Check sheet for the modelled part. Datum: model origin and axes. Units: mm. A direction names the side the tool comes from. Give positions to 0.01 mm unless a question says otherwise; leave off trailing zeros. Loops run counter-clockwise (first coordinate to the right, second up) from the corner with the lowest first, then second, coordinate; pieces in that order, holes last. Notation, with made-up numbers: (55, 76) - (100, 76) arc R22 cw to (100, 114) - close; hole circle Ø6 at (-12.5, -30). An arc over 180 degrees is marked (long way). Use one line per item in the form item = value.
from build123d import *

# Parameters (mm, degrees)
SKETCH_3_W          = 10
SKETCH_3_H          = 3
EXTRUDE_1_DEPTH     = 10
EXTRUDE_1_2_DEPTH   = 10
EXTRUDE_1_3_DEPTH   = 10
EXTRUDE_1_4_DEPTH   = 10
SKETCH_4_W          = 65
SKETCH_4_H          = 9
EXTRUDE_2_DEPTH     = 3
SKETCH_5_R          = 2.1
CUT_EXTRUDE_1_DEPTH = 17
SKETCH_7_W          = 65
SKETCH_7_H          = 3
EXTRUDE_3_DEPTH     = 4
SKETCH_8_W          = 65
SKETCH_8_H          = 3
EXTRUDE_4_DEPTH     = 4


with BuildPart() as part:
    # Sketch 3 → Extrude 1 (new body)
    with BuildSketch(Plane(origin=(0, 0, 0), x_dir=(1, 0, 0), z_dir=(0, 1, 0))):
        Rectangle(SKETCH_3_W, SKETCH_3_H)
    extrude(amount=EXTRUDE_1_DEPTH)



with BuildPart() as body_2:
    # Sketch 3 → Extrude 1 2 (new body)
    with BuildSketch(Plane(origin=(0, 0, 0), x_dir=(1, 0, 0), z_dir=(0, 1, 0))):
        with Locations((55, 0)):
            Rectangle(SKETCH_3_W, SKETCH_3_H)
    extrude(amount=EXTRUDE_1_2_DEPTH)


with BuildPart() as body_3:
    # Sketch 3 → Extrude 1 3 (new body)
    with BuildSketch(Plane(origin=(0, 0, 0), x_dir=(1, 0, 0), z_dir=(0, 1, 0))):
        with Locations((0, 6)):
            Rectangle(SKETCH_3_W, SKETCH_3_H)
    extrude(amount=EXTRUDE_1_3_DEPTH)


with BuildPart() as body_4:
    # Sketch 3 → Extrude 1 4 (new body)
    with BuildSketch(Plane(origin=(0, 0, 0), x_dir=(1, 0, 0), z_dir=(0, 1, 0))):
        with Locations((55, 6)):
            Rectangle(SKETCH_3_W, SKETCH_3_H)
    extrude(amount=EXTRUDE_1_4_DEPTH)


with BuildPart() as part_1:
    add(part.part)

    add(body_2.part)  # Extrude 2 merges body 2

    add(body_3.part)  # Extrude 2 merges body 3

    add(body_4.part)  # Extrude 2 merges body 4
    # Sketch 4 → Extrude 2 (add)
    with BuildSketch(Plane(origin=(0, 10, 0), x_dir=(1, 0, 0), z_dir=(0, 1, 0))):
        with Locations((27.5, 3)):
            Rectangle(SKETCH_4_W, SKETCH_4_H)
    extrude(amount=EXTRUDE_2_DEPTH)

    # Sketch 5 → Cut-Extrude 1 (cut)
    with BuildSketch(Plane.XY.offset(1.5)):
        with Locations((0, 5)):
            Circle(SKETCH_5_R)
        with Locations((55, 5)):
            Circle(SKETCH_5_R)
    extrude(amount=-CUT_EXTRUDE_1_DEPTH, mode=Mode.SUBTRACT)

    # Sketch 7 → Extrude 3 (add)
    with BuildSketch(Plane(origin=(0, 0, -7.5), x_dir=(-1, 0, 0), z_dir=(0, 0, -1))):
        with Locations((-27.5, 11.5)):
            Rectangle(SKETCH_7_W, SKETCH_7_H)
    extrude(amount=EXTRUDE_3_DEPTH)

    # Sketch 8 → Extrude 4 (add)
    with BuildSketch(Plane.XY.offset(1.5)):
        with Locations((27.5, 11.5)):
            Rectangle(SKETCH_8_W, SKETCH_8_H)
    extrude(amount=EXTRUDE_4_DEPTH)


solid = part_1.part
Item 1: Gauge pin test, flat ends, axial feed: P1, Ø1.5, axis at x = 14.5, y = 7.5, coming from the -Z side; P2, Ø3, axis at x = 0.5, y = 7, coming from the -Z side; P3, Ø5, axis at x = -2, y = 5.5, coming from the +Z side. Record the tip position at first contact, or that the pin passes through.
Answer block:
P1 = through
P2 = -7.5
P3 = 1.5
Item 2: Section check A-A on x = 0. Record the boundary of the cut face in (y, z), then the cut area to 3 significant figures.
Answer block:
outline = (0, -7.5) - (2.9, -7.5) - (2.9, -4.5) - (0, -4.5) - close; (0, -1.5) - (2.9, -1.5) - (2.9, 1.5) - (0, 1.5) - close; (7.1, -7.5) - (10, -7.5) - (10, -11.5) - (13, -11.5) - (13, 5.5) - (10, 5.5) - (10, 1.5) - (7.1, 1.5) - (7.1, -1.5) - (10, -1.5) - (10, -4.5) - (7.1, -4.5) - close
area = 85.8 mm2
Item 3: Mould release check, pull along X, two halves, no side actions. Record for faces 6 (the face through (-0.273, 7.082, 0.021)), 7 (the face through (0, 0, -6)): released by +X, released by -X, zero draft, split by the parting line, or undercut.
Answer block:
face_6 = undercut
face_7 = zero draft
Item 4: Thickness scan on L1, parallel to Y at x = 55, z = -6.6; L2, parallel to Z at x = 4.5, y = 6.75; L3, parallel to X at y = 9.25, z = -7. Record the ranges inside material, lowest first.
Answer block:
L1 = 0 to 2.9, 7.1 to 13
L2 = -7.5 to -4.5, -1.5 to 1.5
L3 = -5 to 5, 50 to 60
Item 5: Section check C-C on z = -6.5. Record the boundary of the cut face in (x, y).
Answer block:
outline = (-5, 0) - (5, 0) - (5, 10) - (50, 10) - (50, 0) - (60, 0) - (60, 13) - (-5, 13) - close; hole circle Ø4.2 at (0, 5); hole circle Ø4.2 at (55, 5)
Item 6: Section check B-B on y = 8.5. Record the boundary of the cut face in (x, z).
Answer block:
outline = (-5, -7.5) - (5, -7.5) - (5, -4.5) - (-5, -4.5) - close; (-5, -1.5) - (5, -1.5) - (5, 1.5) - (-5, 1.5) - close; (50, -7.5) - (60, -7.5) - (60, -4.5) - (50, -4.5) - close; (50, -1.5) - (60, -1.5) - (60, 1.5) - (50, 1.5) - close
Item 7: Access from +Z, -Z, +X, -X, +Y, -Y to the whole of each face (thin tool, end or side, straight path). Record for faces 1 (the face through (55, 0, 0)), 2 (the face through (54.9, 2.7, 1.5)), 3 (the face through (-0.1, 2.7, -4.5)), 4 (the face through (50, 5, -6)), 5 (the face through (54.9, 2.7, -7.5)).
Answer block:
face_1 = +Z, -Z, +X, -X, -Y
face_2 = +Z, +X, -X, -Y
face_3 = +X, -X, -Y
face_4 = +Z, -Z, -Y
face_5 = -Z, +X, -X, -Y
Item 8: Section check D-D on y = 5. Give the number of separate pieces and of enclosed holes in the cut face, then the cut area to 3 significant figures.
Answer block:
separate_pieces = 8
enclosed_holes = 0
area = 69.6 mm2
